from build123d import *

# Parameters (mm, degrees)
SKETCH_R              = 20
SKETCH_R_2            = 9
PAD_DEPTH             = 5
POCKET_DEPTH          = 5
POLARPATTERN_COUNT    = 4
PAD001_DEPTH          = 3.5
POLARPATTERN001_COUNT = 5
SKETCH003_R           = 2.7
POCKET001_DEPTH       = 121.431206
POLARPATTERN002_COUNT = 5
SKETCH004_R           = 15
SKETCH004_R_2         = 10.5
POCKET002_DEPTH       = 3
POCKET003_DEPTH       = 5.501
SKETCH006_R           = 2.5
PAD002_DEPTH          = 11.5
POLARPATTERN003_COUNT = 4
SKETCH007_R           = 1.7
POCKET004_DEPTH       = 125.488856
POLARPATTERN004_COUNT = 4


with BuildPart() as part:
    # Sketch → Pad (new body)
    with BuildSketch(Plane.XY):
        Circle(SKETCH_R)
        Circle(SKETCH_R_2, mode=Mode.SUBTRACT)
    extrude(amount=PAD_DEPTH)

    # Sketch001 → Pocket (cut)
    with BuildSketch(Plane.XY.offset(5)):
        with BuildLine():
            Line((3.25, 20), (-3.25, 20))
            ThreePointArc((-3.25, 20), (0, 16.75), (3.25, 20))
        make_face()
    pocket = extrude(amount=-POCKET_DEPTH, mode=Mode.SUBTRACT)

    # PolarPattern: Pocket ×4 about axis
    polarpattern_axis = Axis((0, 0, 5), (0, 0, 1))
    for i in range(1, POLARPATTERN_COUNT):
        add(pocket.rotate(polarpattern_axis, i * 360 / POLARPATTERN_COUNT), mode=Mode.SUBTRACT)

    # Sketch002 → Pad001 (new body)
    with BuildSketch(Plane.XY.offset(5)):
        with BuildLine():
            Line((-4, 16.75), (4, 16.75))
            Line((4, 16.75), (4, 11))
            ThreePointArc((2, 9), (3.414214, 9.585786), (4, 11))
            Line((2, 9), (-2, 9))
            ThreePointArc((-4, 11), (-3.414214, 9.585786), (-2, 9))
            Line((-4, 11), (-4, 16.75))
        make_face()
    pad001 = extrude(amount=PAD001_DEPTH)

    # PolarPattern001: Pad001 ×5 about axis
    polarpattern001_axis = Axis((0, 0, 5), (0, 0, 1))
    for i in range(1, POLARPATTERN001_COUNT):
        add(pad001.rotate(polarpattern001_axis, i * 360 / POLARPATTERN001_COUNT))

    # Sketch003 → Pocket001 (cut, through all)
    with BuildSketch(Plane.XY.offset(8.5)):
        with Locations((0, 12.5)):
            Circle(SKETCH003_R)
    pocket001 = extrude(amount=-POCKET001_DEPTH, mode=Mode.SUBTRACT)

    # PolarPattern002: Pocket001 ×5 about axis
    polarpattern002_axis = Axis((0, 0, 8.5), (0, 0, 1))
    for i in range(1, POLARPATTERN002_COUNT):
        add(pocket001.rotate(polarpattern002_axis, i * 360 / POLARPATTERN002_COUNT), mode=Mode.SUBTRACT)

    # Sketch004 → Pocket002 (cut)
    with BuildSketch(Plane(origin=(0, 0, 0), x_dir=(1, 0, 0), z_dir=(0, 0, -1))):
        Circle(SKETCH004_R)
        Circle(SKETCH004_R_2, mode=Mode.SUBTRACT)
    extrude(amount=-POCKET002_DEPTH, mode=Mode.SUBTRACT)

    # Sketch005 → Pocket003 (cut, through all)
    with BuildSketch(Plane(origin=(0, 0, 3), x_dir=(1, 0, 0), z_dir=(0, 0, -1))):
        with BuildLine():
            ThreePointArc((2.5, 10.198039), (0, 10.5), (-2.5, 10.198039))
            Line((-3.571429, 14.568627), (-2.5, 10.198039))
            ThreePointArc((3.571429, 14.568627), (0, 15), (-3.571429, 14.568627))
            Line((2.5, 10.198039), (3.571429, 14.568627))
        make_face()
    extrude(amount=-POCKET003_DEPTH, mode=Mode.SUBTRACT)

    # Sketch006 → Pad002 (new body)
    with BuildSketch(Plane(origin=(0, 0, 0), x_dir=(1, 0, 0), z_dir=(0, 0, -1))):
        with Locations((-13.435029, 13.435029)):
            Circle(SKETCH006_R)
    pad002 = extrude(amount=-PAD002_DEPTH)

    # PolarPattern003: Pad002 ×4 about axis
    polarpattern003_axis = Axis((0, 0, 0), (0, 0, -1))
    for i in range(1, POLARPATTERN003_COUNT):
        add(pad002.rotate(polarpattern003_axis, i * 360 / POLARPATTERN003_COUNT))

    # Sketch007 → Pocket004 (cut, through all)
    with BuildSketch(Plane(origin=(0, 0, 0), x_dir=(1, 0, 0), z_dir=(0, 0, -1))):
        with Locations((-13.435029, 13.435029)):
            Circle(SKETCH007_R)
    pocket004 = extrude(amount=-POCKET004_DEPTH, mode=Mode.SUBTRACT)

    # PolarPattern004: Pocket004 ×4 about axis
    polarpattern004_axis = Axis((0, 0, 0), (0, 0, -1))
    for i in range(1, POLARPATTERN004_COUNT):
        add(pocket004.rotate(polarpattern004_axis, i * 360 / POLARPATTERN004_COUNT), mode=Mode.SUBTRACT)


solid = part.part
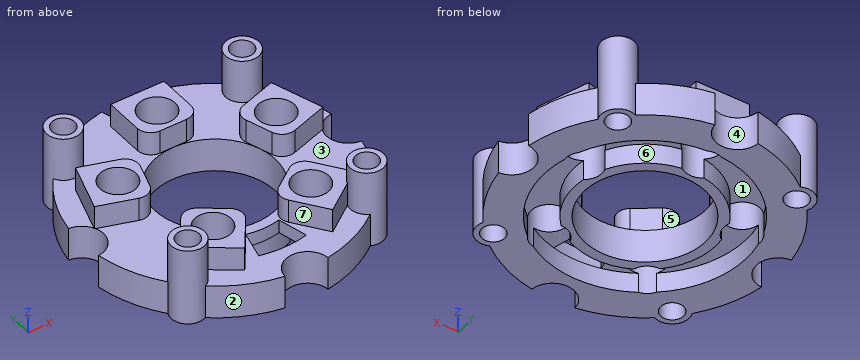
Design review of the part built by this model. Coordinates are the model's own, in mm. Face numbers are marked on the shaded views. A direction names the side the tool comes from. Coordinates: 2 decimals unless noted, no trailing zeros. Order: outer loops, then holes, each group sorted by start corner. A loop starts at its lowest first (then second) coordinate and runs counter-clockwise, first axis right, second up. Notation, with made-up numbers: M 67.25,80 L 109.25,80 A5 cw 109.25,84 Z; hole C 75,72 d9. An arc over 180 degrees is marked long. Use a Markdown table: item, result.
(1) Add section D-D (y = -1.5). Give the boundary of the cut face in (x, z), then the cut area to 3 significant figures.
Worked answers:
| item | result |
|---|---|
| outline | M -17.12,0 L -14.92,0 L -14.92,3 L -10.39,3 L -10.39,0 L -8.87,0 L -8.87,5 L -17.12,5 Z; M 8.87,0 L 10.39,0 L 10.39,3 L 14.92,3 L 14.92,0 L 17.12,0 L 17.12,5 L 8.87,5 Z |
| area | 55.2 mm2 |
(2) Add section A-A (z = 10.25). Give the boundary of the cut face in (x, y).
Worked answers:
| item | result |
|---|---|
| outline | C -13.44,-13.44 d5; C -13.44,13.44 d5; C 13.44,-13.44 d5; C 13.44,13.44 d5; hole C -13.44,-13.44 d3.4; hole C -13.44,13.44 d3.4; hole C 13.44,-13.44 d3.4; hole C 13.44,13.44 d3.4 |
(3) For P1, Ø3, axis at x = -5, y = 12, coming from the -Z side; P2, Ø2, axis at x = 15, z = 6, coming from the -Y side; P3, Ø5, axis at y = 4, z = 8.5, coming from the -X side, all flat-tipped, find the tip position at first contact; note any pin that passes through.
Worked answers:
| item | result |
|---|---|
| P1 | stops at z = 3 |
| P2 | stops at y = -15.87 |
| P3 | stops at x = -17.12 |
(4) Add section C-C (x = -6). Give the boundary of the cut face in (y, z).
Worked answers:
| item | result |
|---|---|
| outline | M -19.08,0 L -13.75,0 L -13.75,3 L -12.45,3 L -12.45,8.5 L -15.06,8.5 L -15.06,5 L -19.08,5 Z; M -7.77,0 L -6.71,0 L -6.71,5 L -6.77,5 L -6.77,8.5 L -7.77,8.5 Z; M 6.71,0 L 8.62,0 L 8.62,3 L 13.75,3 L 13.75,0 L 19.08,0 L 19.08,5 L 6.71,5 Z |
(5) Wall thickness on probe 1 along X at (y, z) = (0, 2.35); probe 2 along X at (y, z) = (4.5, 7.75); probe 3 along Y at (x, z) = (13, 1): over which ranges is each line inside the solid? List them lowest first.
Worked answers:
| item | result |
|---|---|
| probe 1 | x = -16.75 to -15, -10.5 to -9, 9 to 10.5, 15 to 16.75 |
| probe 2 | x = -16.15 to -14.51, -9.26 to -8, 8 to 9.26, 14.51 to 16.15 |
| probe 3 | y = -15.9 to -15.08, -11.79 to -7.48, 7.48 to 11.79, 15.08 to 15.9 |
(6) Draft analysis for pull direction Y (two halves, no side actions). For the marked faces 1, 2, 3 and 4, state which applies: released by +Y, released by -Y, zero draft, split by the parting line, or undercut.
Worked answers:
| item | result |
|---|---|
| face 1 | undercut |
| face 2 | released by -Y |
| face 3 | undercut |
| face 4 | released by +Y |
(7) For the marked faces 5, 6 and 7, list the 3-axis set-ups (+Z, -Z, +X, -X, +Y, -Y) from which the entire face can be reached by the end or side of a thin tool; tool diameter is ignored.
Worked answers:
| item | result |
|---|---|
| face 5 | +Z |
| face 6 | -Z |
| face 7 | +Z, -Y |
(8) Add section B-B (y = 14). Give the boundary of the cut face in (x, z) (3 decimals), then the cut area to 3 significant figures.
Worked answers:
| item | result |
|---|---|
| outline | M -15.87,0 L -15.038,0 L -15.038,11.5 L -15.87,11.5 Z; M -11.832,0 L -5.385,0 L -5.385,3 L -2.245,3 L -2.245,8.5 L -4,8.5 L -4,5 L -11,5 L -11,11.5 L -11.832,11.5 Z; M 2.245,3 L 5.385,3 L 5.385,0 L 11.832,0 L 11.832,11.5 L 11,11.5 L 11,5 L 4,5 L 4,8.5 L 2.245,8.5 Z; M 15.038,0 L 15.87,0 L 15.87,11.5 L 15.038,11.5 Z |
| area | 119 mm2 |
